Build history of the part. All positions in model axes, mm. Face numbers are marked on the shaded views. A direction names the side the tool comes from. Round coordinates to 2 decimals unless told otherwise and drop trailing zeros. Write each loop counter-clockwise with the first axis right and the second up, starting at its lowest first coordinate (ties: lowest second). Pieces come first, ordered by that corner, then holes. Notation, with made-up numbers: M 75,35.5 L 120,35.5 A10 ccw 120,42.5 Z; hole C 22.25,30 d1. An arc over 180 degrees is marked long. Use a Markdown table: item, result.
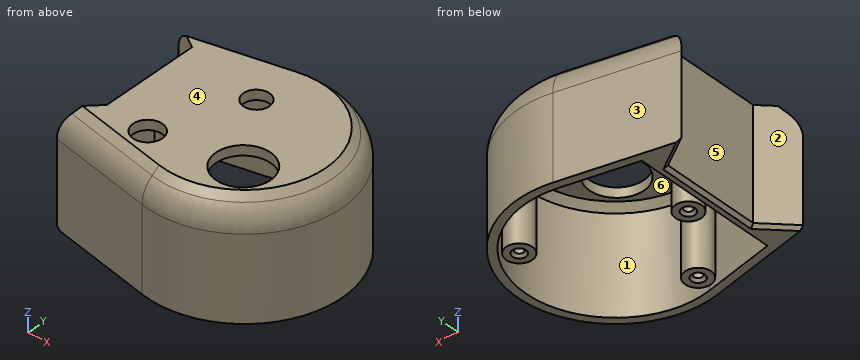
from build123d import *

# Parameters (mm, degrees)
CROQUIS13_R             = 4.5
CROQUIS13_R_2           = 8.4
CROQUIS13_R_3           = 4
SALIENTE_EXTRUIR5_DEPTH = 35
CORTAR_EXTRUIR7_DEPTH   = 32
CHAFL_N6_SIZE           = 5
CHAFL_N7_SIZE           = 2
CROQUIS15_R             = 4
CROQUIS15_R_2           = 1.25
SALIENTE_EXTRUIR9_DEPTH = 32
CHAFL_N8_SIZE           = 0.8
REDONDEO1_R             = 10
CHAFL_N9_SIZE           = 1


with BuildPart() as part:
    # Croquis13 → Saliente-Extruir5 (new body)
    with BuildSketch(Plane.XY):
        with BuildLine():
            Line((-6.126443354, 29.36778323), (-39.789261077, 22.345348329))
            Line((-39.789261077, 22.345348329), (-30, 15.935417314))
            Line((-30, 15.935417314), (-30, -14.387496114))
            Line((-30, -14.387496114), (-38.2739606, -22.661456714))
            Line((-38.2739606, -22.661456714), (-6.126443354, -29.36778323))
            ThreePointArc((-6.126443354, -29.36778323), (30, 0), (-6.126443354, 29.36778323))
        make_face()
        with Locations((-16, -16)):
            Circle(CROQUIS13_R, mode=Mode.SUBTRACT)
        with Locations((10, -12)):
            Circle(CROQUIS13_R_2, mode=Mode.SUBTRACT)
        with Locations((-5, 10)):
            Circle(CROQUIS13_R_3, mode=Mode.SUBTRACT)
    extrude(amount=-SALIENTE_EXTRUIR5_DEPTH)

    # Croquis14 → Cortar-Extruir7 (cut)
    with BuildSketch(Plane(origin=(0, 0, -35), x_dir=(-1, 0, 0), z_dir=(0, 0, -1))):
        with BuildLine():
            Line((27.5, -22.355204771), (5.615906408, -26.920467961))
            ThreePointArc((5.615906408, -26.920467961), (-27.5, 0), (5.615906408, 26.920467961))
            Line((5.615906408, 26.920467961), (27.5, 22.355204771))
            Line((27.5, 22.355204771), (27.5, -22.355204771))
        make_face()
    extrude(amount=-CORTAR_EXTRUIR7_DEPTH, mode=Mode.SUBTRACT)

    # Chaflán6
    chafl_n6_edges = [part.edges().sort_by_distance(p)[0] for p in [
        (-22.200201977, -26.014619972, 0),
        (-22.957852215, 25.856565779, 0),
        (30, 0, 0),
    ]]
    chamfer(chafl_n6_edges, length=CHAFL_N6_SIZE)

    # Chaflán7
    chafl_n7_edges = [part.edges().sort_by_distance(p)[0] for p in [
        (-16.557953204, 24.637836366, -3),
        (27.5, 0, -3),
        (-16.557953204, -24.637836366, -3),
    ]]
    chamfer(chafl_n7_edges, length=CHAFL_N7_SIZE)

    # Croquis15 → Saliente-Extruir9 (add)
    # profile 1 of 3: a face of its own
    with BuildSketch(Plane(origin=(0, 0, -3), x_dir=(-1, 0, 0), z_dir=(0, 0, -1))):
        with Locations(Location((22.5, 0, 0), (0, 0, 180))):
            Circle(CROQUIS15_R)
        with Locations(Location((22.5, 0, 0), (0, 0, 180))):
            Circle(CROQUIS15_R_2, mode=Mode.SUBTRACT)
    # profile 2 of 3: a face of its own
    with BuildSketch(Plane(origin=(0, 0, -3), x_dir=(-1, 0, 0), z_dir=(0, 0, -1))):
        with Locations(Location((6.952882373, -21.398771617, 0), (0, 0, 180))):
            Circle(CROQUIS15_R)
        with Locations(Location((6.952882373, -21.398771617, 0), (0, 0, 180))):
            Circle(CROQUIS15_R_2, mode=Mode.SUBTRACT)
    # profile 3 of 3: a face of its own
    with BuildSketch(Plane(origin=(0, 0, -3), x_dir=(-1, 0, 0), z_dir=(0, 0, -1))):
        with Locations(Location((-18.202882373, 13.225168177, 0), (0, 0, 180))):
            Circle(CROQUIS15_R)
        with Locations(Location((-18.202882373, 13.225168177, 0), (0, 0, 180))):
            Circle(CROQUIS15_R_2, mode=Mode.SUBTRACT)
    extrude(amount=SALIENTE_EXTRUIR9_DEPTH)

    # Chaflán8
    chafl_n8_edges = [part.edges().sort_by_distance(p)[0] for p in [
        (-23.75, 0, -35),
        (-8.202882373, -21.398771617, -35),
        (16.952882373, 13.225168177, -35),
    ]]
    chamfer(chafl_n8_edges, length=CHAFL_N8_SIZE)

    # Redondeo1
    redondeo1_edges = [part.edges().sort_by_distance(p)[0] for p in [
        (-22.957852215, 25.856565779, -5),
        (30, 0, -5),
        (-22.200201977, -26.014619972, -5),
    ]]
    fillet(redondeo1_edges, radius=REDONDEO1_R)

    # Chaflán9
    chafl_n9_edges = [part.edges().sort_by_distance(p)[0] for p in [
        (-34.894630538, 19.140382822, -35),
        (-30, 0.7739606, -35),
        (-34.1369803, -18.524476414, -35),
    ]]
    chamfer(chafl_n9_edges, length=CHAFL_N9_SIZE)


solid = part.part
Q1. Two-plate mould, pull along X, no slides. Class the marked faces 4, 5 and 6: +X half, -X half, draft (parallel to the pull), parting line (faces both ways), or undercut.
Response values:
| item | result |
|---|---|
| face 4 | draft |
| face 5 | -X half |
| face 6 | undercut |
Q2. Drill centre lines: L1, parallel to Y at x = -22.5, z = -8.5; L2, parallel to Y at x = -22, z = -21; L3, parallel to X at y = 14, z = -27.5. Where is each one in solid material? Low to high.
Response values:
| item | result |
|---|---|
| L1 | y = -25.93 to -23.4, -4 to -1.25, 1.25 to 4, 23.4 to 25.93 |
| L2 | y = -26.06 to -23.5, -3.97 to -1.15, 1.15 to 3.97, 23.5 to 26.06 |
| L3 | x = -30 to -27.5, 14.28 to 17.22, 19.18 to 22.13, 23.67 to 26.53 |
Q3. Cut at B-B on y = -16. Count the separate pieces of the cut face and the enclosed holes in it, and give its area (3 significant figures).
Response values:
| item | result |
|---|---|
| separate pieces | 3 |
| enclosed holes | 0 |
| area | 312 mm2 |
Q4. Which spindle directions (+Z, -Z, +X, -X, +Y, -Y) get a long thin tool onto all of the face, cutting with end or side? Do the marked faces 1, 2 and 3. Say none if no direction does.
Response values:
| item | result |
|---|---|
| face 1 | -Z |
| face 2 | +Z, -Z, -X |
| face 3 | +Z, -Z, -X, +Y |
Q5. Cut at A-A on z = -10.5. Give the cut face in (x, y), and give its area (3 significant figures).
Response values:
| item | result |
|---|---|
| outline | M -39.79,22.35 L -30,15.94 L -30,-14.39 L -38.27,-22.66 L -6.13,-29.37 A30 ccw long -6.13,29.37 Z; C -22.5,0 d8; C -6.95,-21.4 d8; C 18.2,13.23 d8; hole M -27.5,-22.36 L -5.62,-26.92 A27.5 ccw long -5.62,26.92 L -27.5,22.36 Z; hole C -22.5,0 d2.5; hole C -6.95,-21.4 d2.5; hole C 18.2,13.23 d2.5 |
| area | 708 mm2 |
Q6. Drop flat-ended pins along their axis: P1, Ø3, axis at x = -22.5, y = 0, coming from the -Z side; P2, Ø1.5, axis at x = -12, y = 8, coming from the -Z side; P3, Ø12, axis at x = -30.5, z = -24, coming from the +Y side. Give the stop position or say it passes through.
Response values:
| item | result |
|---|---|
| P1 | stops at z = -34.45 |
| P2 | stops at z = -3 |
| P3 | stops at y = 25.53 |
